from build123d import *

# Parameters (mm, degrees)
F1_DEPTH = 25
F2_SIZE  = 20
F3_R     = 50


with BuildPart() as f1:
    # F0 (on Top) → F1 (new body)
    with BuildSketch(Plane.XY):
        Polygon((-240, -230), (240, -230), (240, 160), (170, 230), (-170, 230), (-240, 160), align=None)
    extrude(amount=F1_DEPTH)

    # F2
    f2_edges = [f1.edges().sort_by_distance(p)[0] for p in [
        (205, 195, 25),
        (-205, 195, 25),
        (0, 230, 25),
        (240, -35, 25),
        (-240, -35, 25),
        (0, -230, 25),
    ]]
    chamfer(f2_edges, length=F2_SIZE)

    # F3
    f3_edges = [f1.edges().sort_by_distance(p)[0] for p in [
        (0, 210, 25),
        (190.857864, 180.857864, 25),
        (220, -29.142136, 25),
        (-190.857864, 180.857864, 25),
        (-220, -29.142136, 25),
        (0, -210, 25),
    ]]
    fillet(f3_edges, radius=F3_R)


solid = f1.part
Check sheet for the modelled part. Datum: model origin and axes. Units: mm. Give positions to 0.01 mm unless a question says otherwise; leave off trailing zeros. Loops run counter-clockwise (first coordinate to the right, second up) from the corner with the lowest first, then second, coordinate; pieces in that order, holes last. Notation, with made-up numbers: M -6,-13.5 L 32,-13.5 A18 ccw 32,1.5 Z; hole C 14,-8.75 d10. An arc over 180 degrees is marked long. Answer as a JSON object with one key per item and string values. Group by question number.
Q1. Material ranges on line 1 along Y through (x, z) = (-128, 10.25); line 2 along Z through (x, y) = (213.5, -89.5); line 3 along Y through (x, z) = (207, 6.5), recorded low to high. Write a range as [from, to].
Q2. Cross-section at C-C on z = 14.75. Record the cut outline in (x, y), then the cut area to 3 significant figures.
Q3. Go/stop test with flat-tipped pins: P1, Ø4, axis at x = 149.5, y = -171.5, coming from the -Z side; P2, Ø8, axis at x = 169.5, z = 10.5, coming from the +Y side; P3, Ø1.5, axis at y = -28, z = 19.5, coming from the -X side; P4, Ø2, axis at x = -28.5, z = 6.5, coming from the +Y side. Record where each tip stops, or that it passes through.
Q4. Cross-section at A-A on x = -56. Record the cut outline in (y, z).
Q5. Cross-section at B-B on y = 104. Record the cut outline in (x, z).
Evaluation:
{
 "1": {"line 1": "y = [-224.75, 224.75]", "line 2": "z = [0, 22.94]", "line 3": "y = [-228.5, 190.88]"},
 "2": {"outline": "M -229.62,-219.62 L 229.62,-219.62 L 229.62,155.7 L 165.7,219.62 L -165.7,219.62 L -229.62,155.7 Z", "area": "198,000 mm2"},
 "3": {"P1": "stops at z = 0", "P2": "stops at y = 228.5", "P3": "stops at x = -223.5", "P4": "stops at y = 229.5"},
 "4": {"outline": "M -230,0 L 230,0 L 230,5 L 224.64,10.36 A50 ccw 189.29,25 L -189.29,25 A50 ccw -224.64,10.36 L -230,5 Z"},
 "5": {"outline": "M -240,0 L 240,0 L 240,5 L 234.64,10.36 A50 ccw 199.29,25 L -199.29,25 A50 ccw -234.64,10.36 L -240,5 Z"}
}
